Could you check a few things on this model? Use its own coordinates, in mm. Face numbers are marked on the shaded views. A direction names the side the tool comes from. Coordinates: 2 decimals unless noted, no trailing zeros. Write each loop counter-clockwise with the first axis right and the second up, starting at its lowest first coordinate (ties: lowest second). Pieces come first, ordered by that corner, then holes. Notation, with made-up numbers: M 52,41.5 L 93,41.5 A10 ccw 93,55.5 Z; hole C 76.5,54 d7. An arc over 180 degrees is marked long. Answer as CSV lines item,"result". Start each with the question number.
Item 1: I'm going to push flat-ended pins straight in: P1, Ø4, axis at x = -6.5, z = 3, coming from the +Y side; P2, Ø1, axis at x = 7.5, z = 1, coming from the -Y side; P3, Ø12, axis at x = -1.5, y = -1.5, coming from the +Z side; P4, Ø3, axis at x = -2.5, z = 6, coming from the +Y side. Where does each tip first touch, or does it pass through?
Item 2: On a 3-axis mill with a long thin cutter (end or side, diameter ignored), from which of +Z, -Z, +X, -X, +Y, -Y can I reach the whole of each face in a straight line? I mean the marked faces 4 and 5. Say none if no direction works.
Item 3: Suppose I cut it at A-A, the plane y = 0. Write out the boundary of the cut face in (x, z), and give its area (3 significant figures).
Item 4: We'd pull the mould along Y, two halves only. Please class the marked faces 1, 2 and 3: +Y half, -Y half, draft (parallel to the pull), parting line (faces both ways), or undercut.
Item 5: If I drill on line 1 along X through (y, z) = (0, 5.25); line 2 along Y through (x, z) = (4.75, 3), over which ranges is the centre line in solid material (lowest first)? Write a range as [from, to].
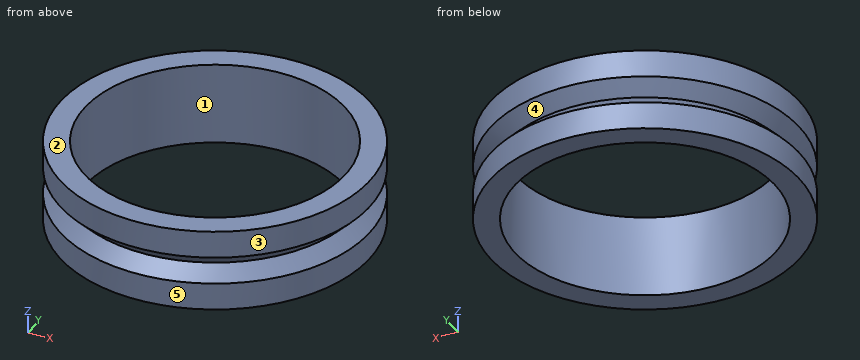
Autodesk Inventor part; units mm, degrees
ref_plane "YZ Plane" through (0, 0, 0) normal (1, 0, 0) x (0, 1, 0)
ref_plane "XZ Plane" through (0, 0, 0) normal (0, 1, 0) x (-1, 0, 0)
ref_plane "XY Plane" through (0, 0, 0) normal (0, 0, 1) x (1, 0, 0)
sketch "Sketch1" plane through (0, 0, 0) normal (0, 1, 0) x (-1, 0, 0)
  line L0 (11.1, 0) -> (11.1, 7)
  line L1 (11.1, 7) -> (13.1667, 7)
  line L2 (13.1667, 7) -> (13.1667, 4.6667)
  line L3 (13.1667, 4.6667) -> (12, 3.5)
  line L4 (12, 3.5) -> (13.1667, 2.3333)
  line L5 (13.1667, 2.3333) -> (13.1667, 0)
  line L6 (13.1667, 0) -> (11.1, 0)
  line L7 (0, 0) -> (0, 4.5986)
  line L8 (13.1667, 4.6667) -> (13.1667, 2.3333)
  dimension "d0" = 11.1
  dimension "d3" = 7
  dimension "d4" = 12
revolve "Revolution1" add sketch "Sketch1" angle 360 about axis through (0, 0, 0) along (0, 0, 1) contours L0 L1 L2 L3 L4 L5 L6
properties part number "z idler"
Ans:
1,P1,"stops at y = 12.33"
1,P2,"stops at y = -11.15"
1,P3,"passes through"
1,P4,"stops at y = 13.13"
2,face 4,"none"
2,face 5,"+Z, -Z"
3,outline,"M -13.17,0 L -11.1,0 L -11.1,7 L -13.17,7 L -13.17,4.67 L -12,3.5 L -13.17,2.33 Z; M 11.1,0 L 13.17,0 L 13.17,2.33 L 12,3.5 L 13.17,4.67 L 13.17,7 L 11.1,7 Z"
3,area,"26.2 mm^2"
4,face 1,"undercut"
4,face 2,"draft"
4,face 3,"parting line"
5,line 1,"x = [-13.17, -11.1], [11.1, 13.17]"
5,line 2,"y = [-11.56, -10.03], [10.03, 11.56]"
